from build123d import *

# Parameters (mm, degrees)
EXTRUIR1_DEPTH      = 20
EXTRUIR2_REACH      = 102.774
EXTRUIR2_END_RADIUS = 33
EXTRUIR2_START      = 50
CROQUIS2_R          = 5
REDONDEO1_R         = 3
REDONDEO2_R         = 1


with BuildPart() as part:
    # Croquis1 → Extruir1 (new body)
    with BuildSketch(Plane(origin=(0, 0, 0), x_dir=(1, 0, 0), z_dir=(0, 1, 0))):
        with BuildLine():
            Line((28.578838325, 16.5), (25.11473671, 14.5))
            ThreePointArc((25.11473671, 14.5), (0, -29), (-25.11473671, 14.5))
            Line((-25.11473671, 14.5), (-28.578838325, 16.5))
            ThreePointArc((-28.578838325, 16.5), (0, -33), (28.578838325, 16.5))
        make_face()
    extrude(amount=EXTRUIR1_DEPTH)

    # Extruir2: up to this cylinder (the profile starts outside it)
    extruir2_end = Plane(origin=(0, 10, 0), z_dir=(0, -1, 0)) * Cylinder(EXTRUIR2_END_RADIUS, 272.548, mode=Mode.PRIVATE)
    # Croquis2 → Extruir2 (add, up to the surface)
    with BuildSketch(Plane.XY.offset(EXTRUIR2_START), mode=Mode.PRIVATE) as extruir2_sk1:
        with Locations((0, 10)):
            Circle(CROQUIS2_R)
    extruir2_tool1 = extrude(extruir2_sk1.sketch, amount=-EXTRUIR2_REACH, mode=Mode.PRIVATE) - extruir2_end
    add(extruir2_tool1.solids().sort_by_distance((0, 10, 50))[0])

    # Redondeo1
    redondeo1_edges = [part.edges().sort_by_distance(p)[0] for p in [
        (25.11473671, 10, -14.5),
        (-25.11473671, 10, -14.5),
    ]]
    fillet(redondeo1_edges, radius=REDONDEO1_R)

    # Redondeo2
    redondeo2_edges = [part.edges().sort_by_distance(p)[0] for p in [
        (0, 20, 33),
        (-28.084798824, 0, -16.214766161),
        (-28.084798824, 20, -16.214766161),
        (0, 0, 29),
        (28.084798824, 0, -16.214766161),
        (26.232610791, 0, -14.243040978),
        (-26.232610791, 0, -14.243040978),
        (0, 20, 29),
        (28.084798824, 20, -16.214766161),
        (26.232610791, 20, -14.243040978),
        (-26.232610791, 20, -14.243040978),
        (0, 0, 33),
        (28.578838325, 10, -16.5),
        (-28.578838325, 10, -16.5),
    ]]
    fillet(redondeo2_edges, radius=REDONDEO2_R)


solid = part.part
Check sheet for the modelled part. Datum: model origin and axes. Units: mm. A direction names the side the tool comes from. Round coordinates to 2 decimals unless told otherwise and drop trailing zeros. Loops run counter-clockwise (first coordinate to the right, second up) from the corner with the lowest first, then second, coordinate; pieces in that order, holes last. Notation, with made-up numbers: M -28,70.25 L -10,70.25 A14 cw -10,77.25 Z; hole C 29.5,43 d4. An arc over 180 degrees is marked long. One line per item, written item: value.
(1) Sectioned sample at B-B, the plane y = 10. Record the cut outline in (x, z).
Computed values:
outline: M -29.08,-15.6 A1 ccw -27.7,-15.99 L -27.59,-15.93 A3 ccw -26.36,-12.08 A29 cw long 26.36,-12.08 A3 ccw 27.59,-15.93 L 27.7,-15.99 A1 ccw 29.08,-15.6 A33 ccw 5,32.62 L 5,50 L -5,50 L -5,32.62 A33 ccw Z
(2) Thickness scan on line 1 (Z direction, x = -26.5, y = 6); line 2 (Z direction, x = -29.5, y = 14.75); line 3 (X direction, y = 18.25, z = 12). Record the ranges inside material, lowest first.
Computed values:
line 1: z = -14.84 to -11.78, 11.78 to 19.67
line 2: z = -14.79 to 14.79
line 3: x = -30.74 to -26.4, 26.4 to 30.74
(3) Depth check by flat-ended pin: pin 1 Ø4 at (x, y) = (-16, 15.5) entering from -Z; pin 2 Ø1.5 at (y, z) = (3.5, 7.5) entering from -X; pin 3 Ø1 at (y, z) = (10.5, 40) entering from +X. Enter the tip coordinate at first touch or a pass-through.
Computed values:
pin 1: stops at z = 22.74
pin 2: stops at x = -32.3
pin 3: stops at x = 5
(4) Sectioned sample at A-A, the plane x = 0. Record the cut outline in (y, z).
Computed values:
outline: M 0,30 A1 ccw 1,29 L 19,29 A1 ccw 20,30 L 20,32 A1 ccw 19,33 L 15,33 L 15,50 L 5,50 L 5,33 L 1,33 A1 ccw 0,32 Z
(5) Sectioned sample at C-C, the plane y = 4. Record the cut outline in (x, z).
Computed values:
outline: M -29.08,-15.6 A1 ccw -27.7,-15.99 L -27.59,-15.93 A3 ccw -26.36,-12.08 A29 cw long 26.36,-12.08 A3 ccw 27.59,-15.93 L 27.7,-15.99 A1 ccw 29.08,-15.6 A33 ccw long Z
(6) Access from +Z, -Z, +X, -X, +Y, -Y to the whole of each face (thin tool, end or side, straight path). Record for faces 1 (the face through (0, 10, 50)), 2 (the face through (-26.223, 10.126, -14.213)), 3 (the face through (-0.651, 14.957, 41.431)).
Computed values:
face 1: +Z, +X, -X, +Y, -Y
face 2: +Y, -Y
face 3: +Z
